Here's how the part is built. I have some questions about the finished solid (model axes, mm). Face numbers are marked on the shaded views. A direction names the side the tool comes from. Coordinates: 2 decimals unless noted, no trailing zeros. Order: outer loops, then holes, each group sorted by start corner. A loop starts at its lowest first (then second) coordinate and runs counter-clockwise, first axis right, second up. Notation, with made-up numbers: (-16, -11.5) - (31, -11.5) arc R18 cw to (31, 17.5) - close; hole circle Ø8 at (55, 31.25). An arc over 180 degrees is marked (long way). Use one line per item in the form item = value. Start each with the question number.
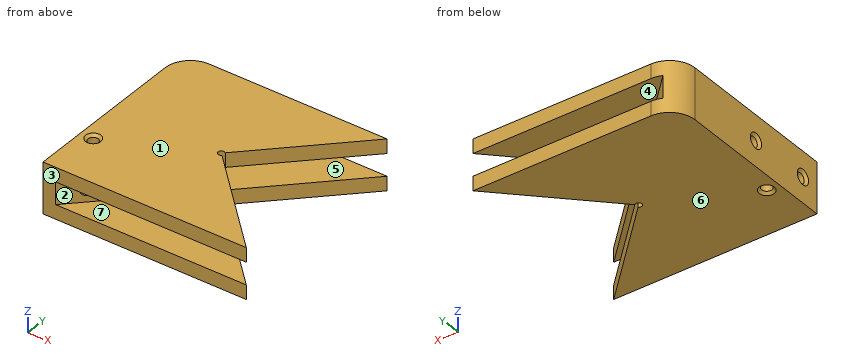
from build123d import *

# Parameters (mm, degrees)
BOSS_EXTRUDE1_DEPTH               = 12.7
F_1_8_0_125_DIAMETER_HOLE1_D      = 3.175
FILLET1_R                         = 12.7
F_1_4_20_TAPPED_HOLE2_D           = 5.1054
F_1_4_20_TAPPED_HOLE2_DEPTH       = 15.875
F_1_4_20_TAPPED_HOLE2_CSINK_D     = 7.62
F_1_4_20_TAPPED_HOLE2_CSINK_ANGLE = 90
F_1_4_20_TAPPED_HOLE2_TIP         = 1.533816902
CUT_EXTRUDE1_DEPTH                = 5.55625


with BuildPart() as part:
    # Sketch2 → Boss-Extrude1 (new, symmetric)
    with BuildSketch(Plane.XY):
        Polygon((0, 0), (0, 95.25), (101.6, 95.25), (53.975, 47.625), (101.6, 0), align=None)
    extrude(amount=BOSS_EXTRUDE1_DEPTH, both=True)

    # 1/8 (0.125) Diameter Hole1 (through all)
    with Locations(Plane.XY.offset(12.7)):
        with Locations((53.975, 47.625)):
            Hole(F_1_8_0_125_DIAMETER_HOLE1_D / 2)

    # Fillet1
    fillet1_edges = [part.edges().sort_by_distance(p)[0] for p in [
        (0, 95.25, 0),
    ]]
    fillet(fillet1_edges, radius=FILLET1_R)

    # Sketch5 → 1/4-20 Tapped Hole1 (revolve, cut)
    with BuildSketch(Plane(origin=(6.35, 25.4, 12.7), x_dir=(0, -1, 0), z_dir=(1, 0, 0))):
        Polygon((0, 0), (0, 25.4), (3.81, 25.4), (2.5527, 24.1427), (2.5527, 1.2573), (3.81, 0), align=None)
    revolve(axis=Axis((6.35, 25.4, 19.05), (0, 0, -1)), mode=Mode.SUBTRACT)

    # 1/4-20 Tapped Hole2
    with Locations(Plane.ZY):
        with Locations((0, 41.275), (0, 9.525)):
            CounterSinkHole(F_1_4_20_TAPPED_HOLE2_D / 2, F_1_4_20_TAPPED_HOLE2_CSINK_D / 2, depth=F_1_4_20_TAPPED_HOLE2_DEPTH, counter_sink_angle=F_1_4_20_TAPPED_HOLE2_CSINK_ANGLE)
            with Locations((0, 0, -(F_1_4_20_TAPPED_HOLE2_DEPTH + F_1_4_20_TAPPED_HOLE2_TIP / 2))):  # 118° drill point
                Cone(0, F_1_4_20_TAPPED_HOLE2_D / 2, F_1_4_20_TAPPED_HOLE2_TIP, mode=Mode.SUBTRACT)

    # Sketch9 → Cut-Extrude1 (cut, symmetric)
    with BuildSketch(Plane.XY):
        Polygon((53.975, 47.625), (101.6, 95.25), (6.35, 95.25), align=None)
        Polygon((101.6, 0), (53.975, 47.625), (6.35, 0), align=None)
    extrude(amount=CUT_EXTRUDE1_DEPTH, both=True, mode=Mode.SUBTRACT)


solid = part.part
1) Suppose I cut it at A-A, the plane x = 61. List the corners of the cut face in (y, z) for me, then the cut area to 3 significant figures.
2) Suppose I cut it at C-C, the plane x = 43. List the corners of the cut face in (y, z) for me, then the cut area to 3 significant figures.
3) Suppose I cut it at D-D, the plane x = 89. List the corners of the cut face in (y, z) for me.
4) Which directions (+Z, -Z, +X, -X, +Y, -Y) give clear straight access to the entire face, cutting with the end or side of a thin tool? Please do the marked faces 5, 6 and 7.
5) Suppose I cut it at B-B, the plane y = 25.4. List the corners of the cut face in (x, z) for me, then the cut area to 3 significant figures.
6) I need wall thicknesses on probe 1 along Z at (x, y) = (77, 79.5); probe 2 along Y at (x, z) = (10.25, 0); probe 3 along Y at (x, z) = (11.75, 0). Which ranges of each line are inside material? Lowest first, please. Write a range as [from, to].
7) If we mould it in two halves opening along Z, with no side actions, what happens to the marked faces 1, 2, 3 and 4? For each: pulls with the +Z half, pulls with the -Z half, needs draft (parallel to the pull), parting line crosses it, or undercut.
8) For pin 1 (3 mm diameter, centred on y = 12.5, z = -1, fed in from -X); pin 2 (10 mm diameter, centred on y = 32, z = -8.5, fed in from +X); pin 3 (2 mm diameter, centred on y = 15.5, z = 6, fed in from +X); pin 4 (10 mm diameter, centred on x = 66, y = 49, fed in from +Z), each with a flat end and sliding along its axis, tell me the tip position at first contact or that it passes through.
From the geometry:
q1.outline = (0, -12.7) - (40.6, -12.7) - (40.6, -5.56) - (0, -5.56) - close; (0, 5.56) - (40.6, 5.56) - (40.6, 12.7) - (0, 12.7) - close; (54.65, -12.7) - (95.25, -12.7) - (95.25, -5.56) - (54.65, -5.56) - close; (54.65, 5.56) - (95.25, 5.56) - (95.25, 12.7) - (54.65, 12.7) - close
q1.area = 1,160 mm2
q2.outline = (0, -12.7) - (95.25, -12.7) - (95.25, -5.56) - (58.6, -5.56) - (58.6, 5.56) - (95.25, 5.56) - (95.25, 12.7) - (0, 12.7) - (0, 5.56) - (36.65, 5.56) - (36.65, -5.56) - (0, -5.56) - close
q2.area = 1,600 mm2
q3.outline = (0, -12.7) - (12.6, -12.7) - (12.6, -5.56) - (0, -5.56) - close; (0, 5.56) - (12.6, 5.56) - (12.6, 12.7) - (0, 12.7) - close; (82.65, -12.7) - (95.25, -12.7) - (95.25, -5.56) - (82.65, -5.56) - close; (82.65, 5.56) - (95.25, 5.56) - (95.25, 12.7) - (82.65, 12.7) - close
q4.face_5 = +X, +Y
q4.face_6 = -Z, +X, -X, +Y, -Y
q4.face_7 = +X, -Y
q5.outline = (0, -12.7) - (2.54, -12.7) - (3.8, -11.44) - (3.8, 11.44) - (2.54, 12.7) - (0, 12.7) - close; (8.9, -11.44) - (10.16, -12.7) - (76.2, -12.7) - (76.2, -5.56) - (31.75, -5.56) - (31.75, 5.56) - (76.2, 5.56) - (76.2, 12.7) - (10.16, 12.7) - (8.9, 11.44) - close
q5.area = 1,310 mm2
q6.probe_1 = [-12.7, -5.56], [5.56, 12.7]
q6.probe_2 = [3.9, 6.97], [12.08, 38.72], [43.83, 91.35]
q6.probe_3 = [5.4, 6.97], [12.08, 38.72], [43.83, 89.85]
q7.face_1 = pulls with the +Z half
q7.face_2 = undercut
q7.face_3 = needs draft
q7.face_4 = undercut
q8.pin_1 = 0
q8.pin_2 = 74.6
q8.pin_3 = 87.1
q8.pin_4 = through
